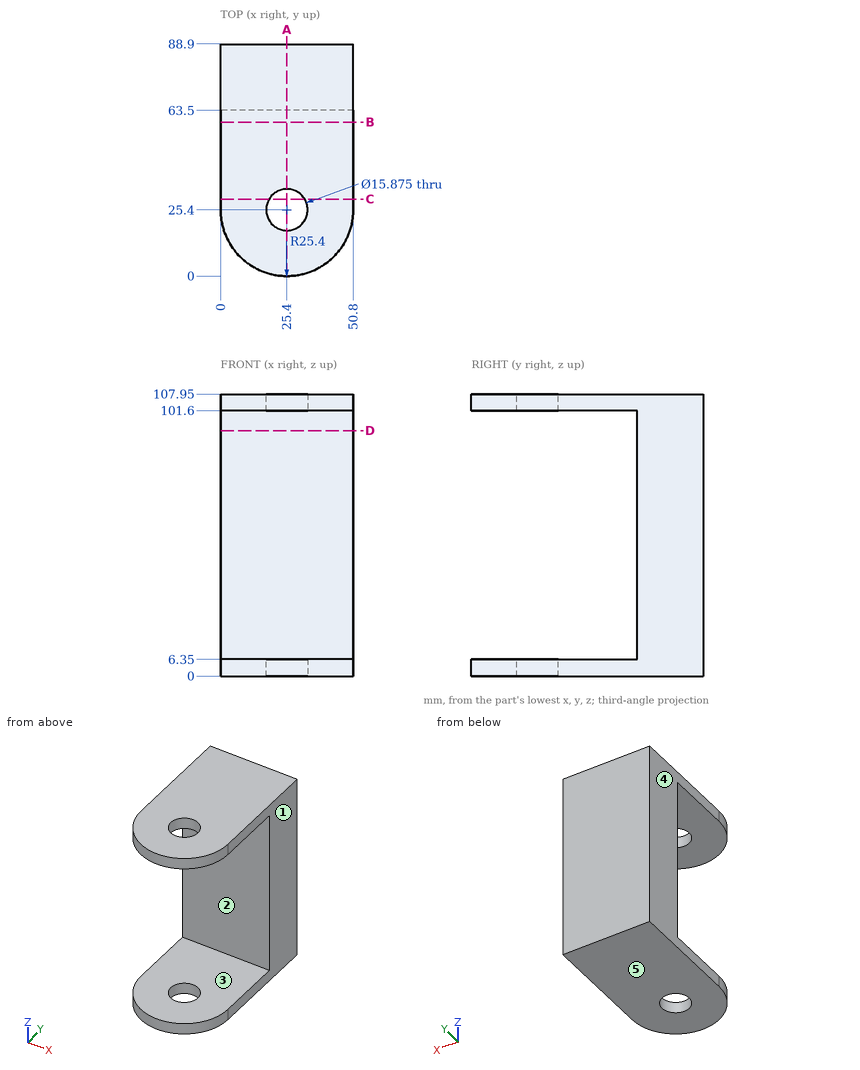
Geometry check sheet. Reference: drawing and pictorial views, mm from the part's lowest x, y, z. A direction names the side the tool comes from. Round coordinates to 2 decimals unless told otherwise and drop trailing zeros. Order: outer loops, then holes, each group sorted by start corner. A loop starts at its lowest first (then second) coordinate and runs counter-clockwise, first axis right, second up. Notation, with made-up numbers: M -24,-18 L -7,-18 A25 cw -7,4 Z; hole C -27,-33 d5. An arc over 180 degrees is marked long. Answer as CSV lines item,"result".
1) Sectioned sample at B-B on y = 59. Record the cut outline in (x, z).
Entries:
outline,"M 0,0 L 50.8,0 L 50.8,6.35 L 0,6.35 Z; M 0,101.6 L 50.8,101.6 L 50.8,107.95 L 0,107.95 Z"
2) Gauge pin test, flat end, axial feed: pin 1 Ø15 at (x, z) = (25.5, 42.5) entering from -Y. Record the tip position at first contact, or that the pin passes through.
Entries:
pin 1,"y = 63.5"
3) Tool access check on the marked faces 1 and 2. Record the directions out of +Z, -Z, +X, -X, +Y, -Y that give a thin tool (end or side, any length) a straight path to the whole face; none if there is none.
Entries:
face 1,"+Z, -Z, +X, +Y, -Y"
face 2,"+X, -X, -Y"
4) Thickness scan on probe 1 along Z at (x, y) = (11, 16); probe 2 along Y at (x, z) = (25.4, 105); probe 3 along Y at (x, z) = (9.5, 34). Record the ranges inside material, lowest first. Write a range as [from, to].
Entries:
probe 1,"[0, 6.35], [101.6, 107.95]"
probe 2,"[0, 17.46], [33.34, 88.9]"
probe 3,"[63.5, 88.9]"
5) Sectioned sample at A-A on x = 25.4. Record the cut outline in (y, z).
Entries:
outline,"M 0,0 L 17.46,0 L 17.46,6.35 L 0,6.35 Z; M 0,101.6 L 17.46,101.6 L 17.46,107.95 L 0,107.95 Z; M 33.34,0 L 88.9,0 L 88.9,107.95 L 33.34,107.95 L 33.34,101.6 L 63.5,101.6 L 63.5,6.35 L 33.34,6.35 Z"
6) Sectioned sample at C-C on y = 29.5. Record the cut outline in (x, z), and give its area (3 significant figures).
Entries:
outline,"M 0,0 L 18.6,0 L 18.6,6.35 L 0,6.35 Z; M 0,101.6 L 18.6,101.6 L 18.6,107.95 L 0,107.95 Z; M 32.2,0 L 50.8,0 L 50.8,6.35 L 32.2,6.35 Z; M 32.2,101.6 L 50.8,101.6 L 50.8,107.95 L 32.2,107.95 Z"
area,"473 mm2"
7) Sectioned sample at D-D on z = 94. Record the cut outline in (x, y), and give its area (3 significant figures).
Entries:
outline,"M 0,63.5 L 50.8,63.5 L 50.8,88.9 L 0,88.9 Z"
area,"1,290 mm2"
8) Mould release check, pull along Z, two halves, no side actions. Record for the marked faces 3, 4 and 5: +Z half, -Z half, draft (parallel to the pull), parting line (faces both ways), or undercut.
Entries:
face 3,"undercut"
face 4,"draft"
face 5,"-Z half"
